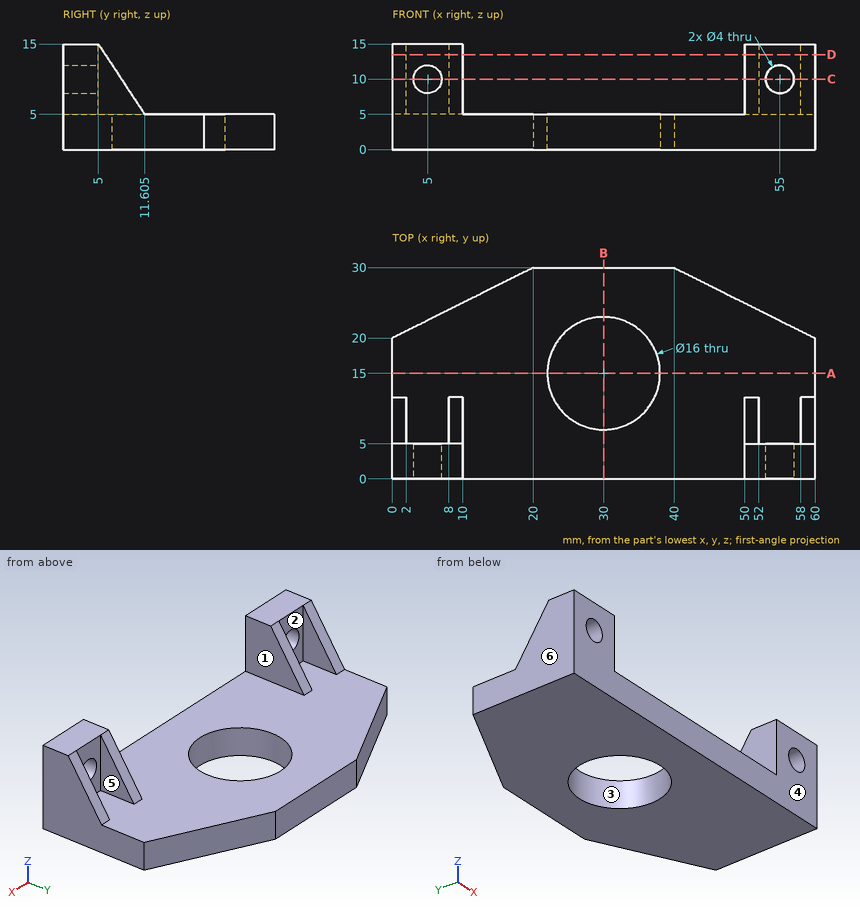
Verification items for this drawing (mm, ordinates from the low corner). A direction names the side the tool comes from. Coordinates: 2 decimals unless noted, no trailing zeros. Write each loop counter-clockwise with the first axis right and the second up, starting at its lowest first coordinate (ties: lowest second). Pieces come first, ordered by that corner, then holes. Notation, with made-up numbers: (0, 2.25) - (36, 2.25) arc R19 ccw to (36, 39.25) - close; hole circle Ø6 at (7, 19). An arc over 180 degrees is marked (long way). One line per question, with ' | ' between items.
Item 1: Sectioned sample at A-A on y = 15. Record the boundary of the cut face in (x, z).
Determined:
outline: (0, 0) - (22, 0) - (22, 5) - (0, 5) - close; (38, 0) - (60, 0) - (60, 5) - (38, 5) - close
Item 2: Mould release check, pull along X, two halves, no side actions. Record for the marked faces 4, 5 and 6: pulls with the +X half, pulls with the -X half, needs draft (parallel to the pull), parting line crosses it, or undercut.
Determined:
face 4: needs draft | face 5: undercut | face 6: pulls with the -X half
Item 3: Sectioned sample at B-B on x = 30. Record the boundary of the cut face in (y, z).
Determined:
outline: (0, 0) - (7, 0) - (7, 5) - (0, 5) - close; (23, 0) - (30, 0) - (30, 5) - (23, 5) - close
Item 4: Gauge pin test, flat ends, axial feed: P1, Ø1.8, axis at x = 55, z = 12, coming from the +Y side; P2, Ø9, axis at x = 35.5, y = 17, coming from the +Z side. Record the tip position at first contact, or that the pin passes through.
Determined:
P1: stops at y = 5 | P2: stops at z = 5
Item 5: Thickness scan on line 1 (Y direction, x = 30, z = 2.75); line 2 (X direction, y = 4.5, z = 7.5); line 3 (Y direction, x = 54, z = 8). Record the ranges inside material, lowest first. Write a range as [from, to].
Determined:
line 1: y = [0, 7], [23, 30] | line 2: x = [0, 10], [50, 60] | line 3: y = [0, 5]
Item 6: Sectioned sample at D-D on z = 13.5. Record the boundary of the cut face in (x, y), plus the area to 3 significant figures.
Determined:
outline: (0, 0) - (10, 0) - (10, 5.99) - (8, 5.99) - (8, 5) - (2, 5) - (2, 5.99) - (0, 5.99) - close; (50, 0) - (60, 0) - (60, 5.99) - (58, 5.99) - (58, 5) - (52, 5) - (52, 5.99) - (50, 5.99) - close | area: 108 mm2
Item 7: Access from +Z, -Z, +X, -X, +Y, -Y to the whole of each face (thin tool, end or side, straight path). Record for the marked faces 1, 2 and 3.
Determined:
face 1: +Z, +Y, -Y | face 2: +Z, +Y | face 3: +Z, -Z
Item 8: Sectioned sample at C-C on z = 10. Record the boundary of the cut face in (x, y).
Determined:
outline: (0, 0) - (3, 0) - (3, 5) - (2, 5) - (2, 8.3) - (0, 8.3) - close; (7, 0) - (10, 0) - (10, 8.3) - (8, 8.3) - (8, 5) - (7, 5) - close; (50, 0) - (53, 0) - (53, 5) - (52, 5) - (52, 8.3) - (50, 8.3) - close; (57, 0) - (60, 0) - (60, 8.3) - (58, 8.3) - (58, 5) - (57, 5) - close
